from build123d import *

# Parameters (mm, degrees)
F1_DEPTH = 1.5
F0_W     = 90
F0_H     = 98
F2_DEPTH = 4
F3_R     = 1
F4_R     = 1.5
F5_DEPTH = 3
F6_R     = 2


with BuildPart() as f1:
    # F0 (on Top) → F1 (new body)
    with BuildSketch(Plane.XY):
        Polygon((43.3765034378, 40.0858414471), (-26.6234965622, 40.0858414471), (-26.6234965622, -37.9141585529), (-2.3734965622, -37.9141585529), (-2.3734965622, -32.9141585529), (19.1265034378, -32.9141585529), (19.1265034378, -37.9141585529), (43.3765034378, -37.9141585529), align=None)
    extrude(amount=F1_DEPTH)

    # F0 (on Top) → F2 (join)
    with BuildSketch(Plane.XY):
        with Locations((8.3765034378, 1.0858414471)):
            Rectangle(F0_W, F0_H)
        with BuildLine():
            ThreePointArc((-31.6234965622, 42.5858414471), (-33.3912635152, 46.8536084001), (-29.1234965622, 45.0858414471))
            Line((-29.1234965622, 45.0858414471), (45.8765034378, 45.0858414471))
            ThreePointArc((45.8765034378, 45.0858414471), (48.3765034378, 47.5858414471), (50.8765034378, 45.0858414471))
            ThreePointArc((50.8765034378, 45.0858414471), (50.1442703907, 43.3180744941), (48.3765034378, 42.5858414471))
            Line((48.3765034378, 42.5858414471), (48.3765034378, -40.4141585529))
            ThreePointArc((48.3765034378, -40.4141585529), (50.1442703907, -41.1463915999), (50.8765034378, -42.9141585529))
            ThreePointArc((50.8765034378, -42.9141585529), (48.3765034378, -45.4141585529), (45.8765034378, -42.9141585529))
            Line((45.8765034378, -42.9141585529), (-29.1234965622, -42.9141585529))
            ThreePointArc((-29.1234965622, -42.9141585529), (-33.3912635152, -44.6819255059), (-31.6234965622, -40.4141585529))
            Line((-31.6234965622, -40.4141585529), (-31.6234965622, 42.5858414471))
        make_face(mode=Mode.SUBTRACT)
        with BuildLine():
            Line((-31.6234965622, -42.9141585529), (-31.6234965622, -40.4141585529))
            ThreePointArc((-31.6234965622, -40.4141585529), (-33.3912635152, -44.6819255059), (-29.1234965622, -42.9141585529))
            Line((-29.1234965622, -42.9141585529), (-31.6234965622, -42.9141585529))
        make_face()
        with BuildLine():
            Line((45.8765034378, 45.0858414471), (-29.1234965622, 45.0858414471))
            ThreePointArc((-29.1234965622, 45.0858414471), (-29.8557296093, 43.3180744941), (-31.6234965622, 42.5858414471))
            Line((-31.6234965622, 42.5858414471), (-31.6234965622, -40.4141585529))
            ThreePointArc((-31.6234965622, -40.4141585529), (-29.8557296093, -41.1463915999), (-29.1234965622, -42.9141585529))
            Line((-29.1234965622, -42.9141585529), (45.8765034378, -42.9141585529))
            ThreePointArc((45.8765034378, -42.9141585529), (46.6087364848, -41.1463915999), (48.3765034378, -40.4141585529))
            Line((48.3765034378, -40.4141585529), (48.3765034378, 42.5858414471))
            ThreePointArc((48.3765034378, 42.5858414471), (46.6087364848, 43.3180744941), (45.8765034378, 45.0858414471))
        make_face()
        Polygon((-26.6234965622, -37.9141585529), (-26.6234965622, 40.0858414471), (43.3765034378, 40.0858414471), (43.3765034378, -37.9141585529), (19.1265034378, -37.9141585529), (-2.3734965622, -37.9141585529), align=None, mode=Mode.SUBTRACT)
        with BuildLine():
            ThreePointArc((-29.1234965622, -42.9141585529), (-29.8557296093, -41.1463915999), (-31.6234965622, -40.4141585529))
            Line((-31.6234965622, -40.4141585529), (-31.6234965622, -42.9141585529))
            Line((-31.6234965622, -42.9141585529), (-29.1234965622, -42.9141585529))
        make_face()
        with BuildLine():
            ThreePointArc((50.8765034378, -42.9141585529), (50.1442703907, -41.1463915999), (48.3765034378, -40.4141585529))
            Line((48.3765034378, -40.4141585529), (48.3765034378, -42.9141585529))
            Line((48.3765034378, -42.9141585529), (45.8765034378, -42.9141585529))
            ThreePointArc((45.8765034378, -42.9141585529), (48.3765034378, -45.4141585529), (50.8765034378, -42.9141585529))
        make_face()
        with BuildLine():
            Line((48.3765034378, -42.9141585529), (48.3765034378, -40.4141585529))
            ThreePointArc((48.3765034378, -40.4141585529), (46.6087364848, -41.1463915999), (45.8765034378, -42.9141585529))
            Line((45.8765034378, -42.9141585529), (48.3765034378, -42.9141585529))
        make_face()
        with BuildLine():
            Line((48.3765034378, 45.0858414471), (45.8765034378, 45.0858414471))
            ThreePointArc((45.8765034378, 45.0858414471), (46.6087364848, 43.3180744941), (48.3765034378, 42.5858414471))
            Line((48.3765034378, 42.5858414471), (48.3765034378, 45.0858414471))
        make_face()
        with BuildLine():
            ThreePointArc((50.8765034378, 45.0858414471), (48.3765034378, 47.5858414471), (45.8765034378, 45.0858414471))
            Line((45.8765034378, 45.0858414471), (48.3765034378, 45.0858414471))
            Line((48.3765034378, 45.0858414471), (48.3765034378, 42.5858414471))
            ThreePointArc((48.3765034378, 42.5858414471), (50.1442703907, 43.3180744941), (50.8765034378, 45.0858414471))
        make_face()
        with BuildLine():
            Line((-31.6234965622, 42.5858414471), (-31.6234965622, 45.0858414471))
            Line((-31.6234965622, 45.0858414471), (-29.1234965622, 45.0858414471))
            ThreePointArc((-29.1234965622, 45.0858414471), (-33.3912635152, 46.8536084001), (-31.6234965622, 42.5858414471))
        make_face()
        with BuildLine():
            Line((-29.1234965622, 45.0858414471), (-31.6234965622, 45.0858414471))
            Line((-31.6234965622, 45.0858414471), (-31.6234965622, 42.5858414471))
            ThreePointArc((-31.6234965622, 42.5858414471), (-29.8557296093, 43.3180744941), (-29.1234965622, 45.0858414471))
        make_face()
    extrude(amount=F2_DEPTH)

    # F3
    f3_edges = [f1.edges().sort_by_distance(p)[0] for p in [
        (8.376503, -32.914159, 1.5),
        (-26.623497, 1.085841, 4),
        (8.376503, -37.914159, 4),
        (43.376503, 1.085841, 4),
        (8.376503, 40.085841, 4),
    ]]
    fillet(f3_edges, radius=F3_R)

    # F4
    f4_edges = [f1.edges().sort_by_distance(p)[0] for p in [
        (-36.623497, 1.085841, 4),
        (8.376503, 50.085841, 4),
        (53.376503, 1.085841, 4),
        (8.376503, -47.914159, 4),
    ]]
    fillet(f4_edges, radius=F4_R)

    # F0 (on Top) → F5 (cut)
    with BuildSketch(Plane.XY):
        with BuildLine():
            Line((48.3765034378, 45.0858414471), (45.8765034378, 45.0858414471))
            ThreePointArc((45.8765034378, 45.0858414471), (46.6087364848, 43.3180744941), (48.3765034378, 42.5858414471))
            Line((48.3765034378, 42.5858414471), (48.3765034378, 45.0858414471))
        make_face()
        with BuildLine():
            ThreePointArc((50.8765034378, 45.0858414471), (48.3765034378, 47.5858414471), (45.8765034378, 45.0858414471))
            Line((45.8765034378, 45.0858414471), (48.3765034378, 45.0858414471))
            Line((48.3765034378, 45.0858414471), (48.3765034378, 42.5858414471))
            ThreePointArc((48.3765034378, 42.5858414471), (50.1442703907, 43.3180744941), (50.8765034378, 45.0858414471))
        make_face()
        with BuildLine():
            Line((-31.6234965622, 42.5858414471), (-31.6234965622, 45.0858414471))
            Line((-31.6234965622, 45.0858414471), (-29.1234965622, 45.0858414471))
            ThreePointArc((-29.1234965622, 45.0858414471), (-33.3912635152, 46.8536084001), (-31.6234965622, 42.5858414471))
        make_face()
        with BuildLine():
            Line((-29.1234965622, 45.0858414471), (-31.6234965622, 45.0858414471))
            Line((-31.6234965622, 45.0858414471), (-31.6234965622, 42.5858414471))
            ThreePointArc((-31.6234965622, 42.5858414471), (-29.8557296093, 43.3180744941), (-29.1234965622, 45.0858414471))
        make_face()
        with BuildLine():
            Line((48.3765034378, -42.9141585529), (48.3765034378, -40.4141585529))
            ThreePointArc((48.3765034378, -40.4141585529), (46.6087364848, -41.1463915999), (45.8765034378, -42.9141585529))
            Line((45.8765034378, -42.9141585529), (48.3765034378, -42.9141585529))
        make_face()
        with BuildLine():
            ThreePointArc((50.8765034378, -42.9141585529), (50.1442703907, -41.1463915999), (48.3765034378, -40.4141585529))
            Line((48.3765034378, -40.4141585529), (48.3765034378, -42.9141585529))
            Line((48.3765034378, -42.9141585529), (45.8765034378, -42.9141585529))
            ThreePointArc((45.8765034378, -42.9141585529), (48.3765034378, -45.4141585529), (50.8765034378, -42.9141585529))
        make_face()
        with BuildLine():
            Line((-31.6234965622, -42.9141585529), (-31.6234965622, -40.4141585529))
            ThreePointArc((-31.6234965622, -40.4141585529), (-33.3912635152, -44.6819255059), (-29.1234965622, -42.9141585529))
            Line((-29.1234965622, -42.9141585529), (-31.6234965622, -42.9141585529))
        make_face()
        with BuildLine():
            ThreePointArc((-29.1234965622, -42.9141585529), (-29.8557296093, -41.1463915999), (-31.6234965622, -40.4141585529))
            Line((-31.6234965622, -40.4141585529), (-31.6234965622, -42.9141585529))
            Line((-31.6234965622, -42.9141585529), (-29.1234965622, -42.9141585529))
        make_face()
    extrude(amount=F5_DEPTH, mode=Mode.SUBTRACT)

    # F6
    f6_edges = [f1.edges().sort_by_distance(p)[0] for p in [
        (50.876503, -42.914159, 3),
        (48.376503, 47.585841, 3),
        (-31.623497, 47.585841, 3),
        (-34.123497, -42.914159, 3),
    ]]
    fillet(f6_edges, radius=F6_R)


solid = f1.part
Here's how the part is built. I have some questions about the finished solid (model axes, mm). A direction names the side the tool comes from. Coordinates: 2 decimals unless noted, no trailing zeros. Write each loop counter-clockwise with the first axis right and the second up, starting at its lowest first coordinate (ties: lowest second). Pieces come first, ordered by that corner, then holes. Notation, with made-up numbers: (-2, 36) - (2, 36) arc R15 cw to (2, 58) - close; hole circle Ø4 at (-28, 23). An arc over 180 degrees is marked (long way). Use one line per item in the form item = value.
1) Suppose I cut it at B-B, the plane y = 16.5. Write out the boundary of the cut face in (x, z), plus the area to 3 significant figures.
Solved:
outline = (-36.62, 0) - (53.38, 0) - (53.38, 2.5) arc R1.5 ccw to (51.88, 4) - (44.38, 4) arc R1 ccw to (43.38, 3) - (43.38, 1.5) - (-26.62, 1.5) - (-26.62, 3) arc R1 ccw to (-27.62, 4) - (-35.12, 4) arc R1.5 ccw to (-36.62, 2.5) - close
area = 184 mm2
2) Suppose I cut it at C-C, the plane x = 34. Write out the boundary of the cut face in (y, z).
Solved:
outline = (-47.91, 0) - (50.09, 0) - (50.09, 2.5) arc R1.5 ccw to (48.59, 4) - (41.09, 4) arc R1 ccw to (40.09, 3) - (40.09, 1.5) - (-37.91, 1.5) - (-37.91, 3) arc R1 ccw to (-38.91, 4) - (-46.41, 4) arc R1.5 ccw to (-47.91, 2.5) - close
3) On a 3-axis mill with a long thin cutter (end or side, diameter ignored), from which of +Z, -Z, +X, -X, +Y, -Y can I reach the whole of each face in a straight line? I mean faces 1 (the flat face through (8, 2, 1.5)), 2 (the flat face through (-36.623, 0, 1)). Say none if no direction works.
Solved:
face_1 = +Z
face_2 = +Z, -Z, -X, +Y, -Y
4) Suppose I cut it at A-A, the plane x = 10. Write out the boundary of the cut face in (y, z), plus the area to 3 significant figures.
Solved:
outline = (-47.91, 0) - (-37.91, 0) - (-37.91, 3) arc R1 ccw to (-38.91, 4) - (-46.41, 4) arc R1.5 ccw to (-47.91, 2.5) - close; (-32.91, 0) - (50.09, 0) - (50.09, 2.5) arc R1.5 ccw to (48.59, 4) - (41.09, 4) arc R1 ccw to (40.09, 3) - (40.09, 1.5) - (-31.91, 1.5) arc R1 ccw to (-32.91, 0.5) - close
area = 188 mm2
5) I need wall thicknesses on line 1 (X direction, y = 32, z = 2); line 2 (Y direction, x = 40.5, z = 2.3); line 3 (X direction, y = -36.5, z = 1.4). Which ranges of each line are inside material? Lowest first, please.
Solved:
line_1 = -36.62 to -26.62, 43.38 to 53.38
line_2 = -47.91 to -37.91, 40.09 to 50.09
line_3 = -36.62 to -2.37, 19.13 to 53.38
6) I'm going to push flat-ended pins straight in: P1, Ø1.1, axis at x = -31.5, y = -43, coming from the -Z side; P2, Ø8, axis at x = 42.5, y = 2, coming from the -Z side; P3, Ø1.5, axis at x = 8, y = 13.5, coming from the +Z side. Where does each tip first touch, or does it pass through?
Solved:
P1 = 2.99
P2 = 0
P3 = 1.5
